Part model, mm, in its own coordinate system. A direction names the side the tool comes from. Give positions to 0.01 mm unless a question says otherwise; leave off trailing zeros. Order: outer loops, then holes, each group sorted by start corner. A loop starts at its lowest first (then second) coordinate and runs counter-clockwise, first axis right, second up. Notation, with made-up numbers: M 87.5,44 L 135.5,44 A17 cw 135.5,52 Z; hole C 40.5,-18 d2. An arc over 180 degrees is marked long. Return JSON: item names as keys, results as strings.
from build123d import *

# Parameters (mm, degrees)
F0_R         = 1
F1_DEPTH     = 5
F3_DEPTH     = 8
F5_DEPTH     = 1
F6_R         = 1
F7_DEPTH     = 7
F8_R         = 1.75
F9_DEPTH     = 8
F10_R        = 3
F11_DEPTH    = 23.501
F12_W        = 9
F12_H        = 9
F12_R        = 1.95
F13_DEPTH    = 2.5
F16_DEPTH    = 6.5
F17_DEPTH    = 7
F18_R        = 1.75
F19_DEPTH    = 28.001
F20_T2_ANGLE = 180
F20_T4_ANGLE = 63.0666087428
F20_T6_ANGLE = 177.2059132033
F20_T8_ANGLE = 63.0666087428


# Not quite as in the source:
# - a fillet or chamfer that OpenCascade refuses, or shapes differently, is made with other operations: its cross-section is extruded or revolved along the edge and cut away or added


with BuildPart() as f1:
    # F0 (on Top) → F1 (new body, symmetric)
    with BuildSketch(Plane.XY):
        with BuildLine():
            ThreePointArc((-26.3391343821, 9.5), (-24.2249616205, 4.9575872166), (-23.5, 0))
            ThreePointArc((-23.5, 0), (0, -23.5), (23.5, 0))
            ThreePointArc((23.5, 0), (24.2249616205, 4.9575872166), (26.3391343821, 9.5))
            ThreePointArc((26.3391343821, 9.5), (0, 28), (-26.3391343821, 9.5))
        make_face()
        with Locations((-18.5, 0)):
            Circle(F0_R, mode=Mode.SUBTRACT)
        with Locations((18.5, 0)):
            Circle(F0_R, mode=Mode.SUBTRACT)
    extrude(amount=F1_DEPTH, both=True)

    # F2 (on face) → F3 (cut)
    with BuildSketch(Plane(origin=(0, 0, -5), x_dir=(1, 0, 0), z_dir=(0, 0, -1))):
        with BuildLine():
            ThreePointArc((21.5, 0), (0, 21.5), (-21.5, 0))
            ThreePointArc((-21.5, 0), (-22.1675592341, -5.0230125511), (-24.12389255, -9.6973093298))
            ThreePointArc((-24.12389255, -9.6973093298), (0, -26), (24.12389255, -9.6973093298))
            ThreePointArc((24.12389255, -9.6973093298), (22.1675592341, -5.023012551), (21.5, 0))
        make_face()
    extrude(amount=-F3_DEPTH, mode=Mode.SUBTRACT)

    # F4 (on face) → F5 (cut)
    with BuildSketch(Plane(origin=(0, 0, -5), x_dir=(1, 0, 0), z_dir=(0, 0, -1))):
        with BuildLine():
            ThreePointArc((22.7, 0), (0, 22.7), (-22.7, 0))
            ThreePointArc((-22.7, 0), (-23.4028138558, -4.9851365308), (-25.4564681735, -9.5816610319))
            ThreePointArc((-25.4564681735, -9.5816610319), (0, -27.2), (25.4564681736, -9.5816610318))
            ThreePointArc((25.4564681736, -9.5816610318), (23.4028138558, -4.9851365307), (22.7, 0))
        make_face()
    extrude(amount=-F5_DEPTH, mode=Mode.SUBTRACT)

    # F6 (on face) → F7 (join, through all)
    with BuildSketch(Plane(origin=(0, 0, 3), x_dir=(1, 0, 0), z_dir=(0, 0, -1))):
        with BuildLine():
            ThreePointArc((-17.6723561014, -2.888314352), (-15.4992475751, 0.1511261164), (-17.9667347728, 2.9568534655))
            ThreePointArc((-17.9667347728, 2.9568534655), (-20.0762140714, 4.428973477), (-20.3324952956, 6.9885359735))
            ThreePointArc((-20.3324952956, 6.9885359735), (-22.8497447738, -0.1109553271), (-23.0826374703, -7.6399049653))
            ThreePointArc((-23.0826374703, -7.6399049653), (-20.9107637858, -4.6569183518), (-17.6723561014, -2.888314352))
        make_face()
        with Locations((-18.5, 0)):
            Circle(F6_R, mode=Mode.SUBTRACT)
        with BuildLine():
            ThreePointArc((20.3324952956, 6.9885359735), (20.0762140714, 4.428973477), (17.9667347728, 2.9568534655))
            ThreePointArc((17.9667347728, 2.9568534655), (15.4992475751, 0.1511261164), (17.6723561014, -2.888314352))
            ThreePointArc((17.6723561014, -2.888314352), (20.9107637858, -4.6569183518), (23.0826374703, -7.6399049653))
            ThreePointArc((23.0826374703, -7.6399049653), (22.9151781731, -0.0986538692), (20.3324952956, 6.9885359735))
        make_face()
        with Locations((18.5, 0)):
            Circle(F6_R, mode=Mode.SUBTRACT)
    extrude(amount=F7_DEPTH)

    # F8 (on face) → F9 (cut)
    with BuildSketch(Plane.XY.offset(5)):
        with Locations((-18.5, 0)):
            Circle(F8_R)
        with Locations((18.5, 0)):
            Circle(F8_R)
    extrude(amount=-F9_DEPTH, mode=Mode.SUBTRACT)

    # F10 (on Front) → F11 (cut, through all)
    with BuildSketch(Plane.XZ):
        with Locations((0, -5)):
            Circle(F10_R)
    extrude(amount=F11_DEPTH, mode=Mode.SUBTRACT)

    # F12 (on Front) → F13 (join, symmetric)
    with BuildSketch(Plane.XZ):
        with Locations((0, 9.5)):
            Rectangle(F12_W, F12_H)
        with Locations((0, 9.5)):
            Circle(F12_R, mode=Mode.SUBTRACT)
    extrude(amount=F13_DEPTH, both=True)

    # F15 (on face) → F16 (join)
    with BuildSketch(Plane(origin=(0, 0, -4), x_dir=(1, 0, 0), z_dir=(0, 0, -1))):
        with BuildLine():
            ThreePointArc((10.5675868988, -20.9899048863), (0, -23.5), (-10.5675868988, -20.9899048863))
            ThreePointArc((-10.5675868988, -20.9899048863), (-13.6551032171, -20.8795666046), (-15.75, -23.1503239718))
            ThreePointArc((-15.75, -23.1503239718), (0, -28), (15.75, -23.1503239718))
            ThreePointArc((15.75, -23.1503239718), (13.6551032171, -20.8795666046), (10.5675868988, -20.9899048863))
        make_face()
    extrude(amount=F16_DEPTH)

    # F15 (on face) → F17 (join, through all)
    with BuildSketch(Plane(origin=(0, 0, -4), x_dir=(1, 0, 0), z_dir=(0, 0, -1))):
        with BuildLine():
            ThreePointArc((10.5675868988, -20.9899048863), (0, -23.5), (-10.5675868988, -20.9899048863))
            ThreePointArc((-10.5675868988, -20.9899048863), (-13.6551032171, -20.8795666046), (-15.75, -23.1503239718))
            ThreePointArc((-15.75, -23.1503239718), (0, -28), (15.75, -23.1503239718))
            ThreePointArc((15.75, -23.1503239718), (13.6551032171, -20.8795666046), (10.5675868988, -20.9899048863))
        make_face()
    extrude(amount=-F17_DEPTH)

    # F18 (on Front) → F19 (cut, through all)
    with BuildSketch(Plane.XZ):
        with Locations((0, -7.75)):
            Circle(F18_R)
    extrude(amount=-F19_DEPTH, mode=Mode.SUBTRACT)

    # F20: chamfer of 3.5 on 4 edges, made by hand

    # F20_s1 → F20_t2 (revolve, cut)
    with BuildSketch(Plane.XZ):
        Polygon((-20, 5), (-23.5, 1.5), (-23.5, 5), align=None)
    revolve(axis=Axis((0, 0, 5), (0, 0, 1)), revolution_arc=F20_T2_ANGLE, mode=Mode.SUBTRACT)

    # F20_s3 → F20_t4 (revolve, cut)
    with BuildSketch(Plane.XZ):
        Polygon((23.5, 1.5), (20, 5), (23.5, 5), align=None)
    revolve(axis=Axis((40.8134960885, 0, 5), (0, 0, -1)), revolution_arc=F20_T4_ANGLE, mode=Mode.SUBTRACT)

    # F20_s5 → F20_t6 (revolve, cut)
    with BuildSketch(Plane(origin=(0, 0, 0), x_dir=(0, 0, 1), z_dir=(0.0243805911, -0.9997027492, 0))):
        Polygon((1.5, -28), (5, -24.5), (5, -28), align=None)
    revolve(axis=Axis((0, 0, 5), (0, 0, 1)), revolution_arc=F20_T6_ANGLE, mode=Mode.SUBTRACT)

    # F20_s7 → F20_t8 (revolve, cut)
    with BuildSketch(Plane(origin=(-32.4398868868, 16.4814724869, 0), x_dir=(0, 0, 1), z_dir=(-0.8915337049, 0.4529543608, 0))):
        Polygon((5, 2.326845056), (1.5, -1.173154944), (5, -1.173154944), align=None)
    revolve(axis=Axis((-40.8134960885, 0, 5), (0, 0, -1)), revolution_arc=F20_T8_ANGLE, mode=Mode.SUBTRACT)


solid = f1.part
Q1. Two-plate mould, pull along X, no slides. Class faces 5 (the conical face through (0.423, 24.666, 4.83)), 6 (the cylindrical face through (-23.383, 4.917, -4.507)), 7 (the flat face through (4.5, 0, 9)): +X half, -X half, draft (parallel to the pull), parting line (faces both ways), or undercut.
Established:
{"face 5": "parting line", "face 6": "undercut", "face 7": "+X half"}
Q2. Probe line 1 along Z through (x, y) = (0, 25); line 2 along X through (y, z) = (-1.5, 0.5); line 3 along Y through (x, z) = (-18.5, -0.75). List the from-to ranges inside material, lowest first.
Established:
{"line 1": "z = -10.5 to -9.5, -6 to 4.5", "line 2": "x = -23.45 to -19.4, -17.6 to -15.9, 15.9 to 17.6, 19.4 to 23.45", "line 3": "y = -14.49 to -10.95, -3.1 to -1.75, 1.75 to 3.17, 18.27 to 21.02"}
Q3. Pin check, flat tips, straight feed: pin 1 (4 mm diameter, centred on y = 2.5, z = 0.5, fed in from +X) (3 decimals); pin 2 (10 mm diameter, centred on x = 1.5, z = 11, fed in from +Y); pin 3 (3 mm diameter, centred on x = 0, z = -7.75, fed in from -Y); pin 4 (5.5 mm diameter, centred on x = 18.5, y = 0, fed in from -Z). Stop position of each tip, or through.
Established:
{"pin 1": "stops at x = 24.095", "pin 2": "stops at y = 2.5", "pin 3": "passes through", "pin 4": "stops at z = -4"}
Q4. 3-axis set-ups, long thin cutter, end or side, ignore diameter. For faces 1 (the cylindrical face through (17.17, -14.85, -4.51)), 2 (the flat face through (20, 0, -3)), 3 (the cylindrical face through (0, -22, -2)), 4 (the flat face through (-4.5, 0, 9)): which of +Z, -Z, +X, -X, +Y, -Y reach the whole face in a straight line?
Established:
{"face 1": "-Z", "face 2": "+Z", "face 3": "-Z, -Y", "face 4": "+Z, -X, +Y, -Y"}
Q5. Band-saw the part on B-B (z = 8.75). Give the cut face in (x, y).
Established:
{"outline": "M -4.5,-2.5 L -1.8,-2.5 L -1.8,2.5 L -4.5,2.5 Z; M 1.8,-2.5 L 4.5,-2.5 L 4.5,2.5 L 1.8,2.5 Z"}
Q6. Band-saw the part on A-A (x = 0). Give the cut face in (y, z).
Established:
{"outline": "M -23.5,-2 L -21.5,-2 L -21.5,3 L 23.5,3 L 23.5,-6 L 28,-6 L 28,1.5 L 24.5,5 L 2.5,5 L 2.5,7.55 L -2.5,7.55 L -2.5,5 L -20,5 L -23.5,1.5 Z; M -2.5,11.45 L 2.5,11.45 L 2.5,14 L -2.5,14 Z; M 23.5,-10.5 L 28,-10.5 L 28,-9.5 L 23.5,-9.5 Z"}
